For this review, take the finished solid that the model builds, in its own axes (mm). Face numbers are marked on the shaded views. A direction names the side the tool comes from. Give positions to 0.01 mm unless a question says otherwise; leave off trailing zeros. Order: outer loops, then holes, each group sorted by start corner. A loop starts at its lowest first (then second) coordinate and runs counter-clockwise, first axis right, second up.
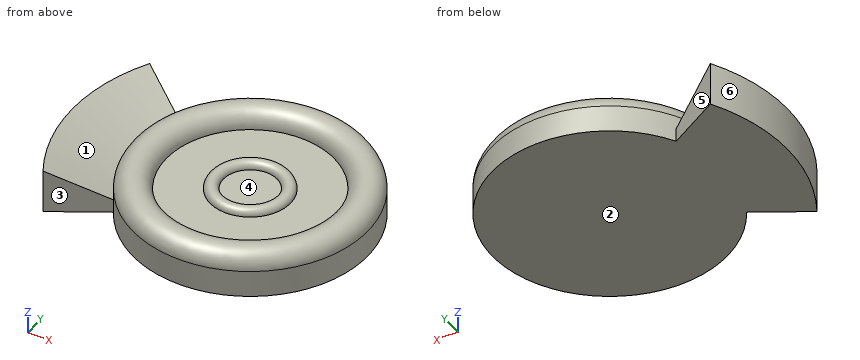
from build123d import *

# Parameters (mm, degrees)
F2_ANGLE = 60


with BuildPart() as f1:
    # F0 (on Front) → F1 (revolve)
    with BuildSketch(Plane.XZ):
        with BuildLine():
            Line((0, -8), (0, 0))
            Line((0, 0), (-8, 0))
            Line((-8, 0), (-12, 0))
            Line((-12, 0), (-25, 0))
            ThreePointArc((-25, 0), (-30, 5), (-35, 0))
            Line((-35, 0), (-35, -4))
            Line((-35, -4), (-35, -8))
            Line((-35, -8), (0, -8))
        make_face()
        with BuildLine():
            Line((-12, 0), (-8, 0))
            ThreePointArc((-8, 0), (-10, 2), (-12, 0))
        make_face()
    revolve(axis=Axis((0, 0, -4), (0, 0, -1)))

    # F0 (on Front) → F2 (revolve, symmetric)
    with BuildSketch(Plane.XZ) as f2_sk:
        Polygon((-53, -8), (-35, -8), (-35, -4), (-53, 5), align=None)
    revolve(axis=Axis((0, 0, -4), (0, 0, -1)), revolution_arc=F2_ANGLE / 2)
    revolve(f2_sk.sketch, axis=Axis((0, 0, -4), (0, 0, 1)), revolution_arc=F2_ANGLE / 2)


solid = f1.part
1) We need section A-A on x = 0. Give the boundary of the cut face in (y, z).
Answer sheet:
outline: (-35, -8) - (35, -8) - (35, 0) arc R5 ccw to (25, 0) - (12, 0) arc R2 ccw to (8, 0) - (-8, 0) arc R2 ccw to (-12, 0) - (-25, 0) arc R5 ccw to (-35, 0) - close
2) We need section B-B on y = 0. Give the boundary of the cut face in (x, z), then the cut area to 3 significant figures.
Answer sheet:
outline: (-53, -8) - (35, -8) - (35, 0) arc R5 ccw to (25, 0) - (12, 0) arc R2 ccw to (8, 0) - (-8, 0) arc R2 ccw to (-12, 0) - (-25, 0) arc R5 ccw to (-35, 0) - (-35, -4) - (-53, 5) - close
area: 804 mm2
3) Clearance check with flat-ended pins moving along their axes: pin 1 (6 mm diameter, centred on x = 19.5, z = 0, fed in from -Y); pin 2 (1 mm diameter, centred on x = -26, y = -3, fed in from +Z); pin 3 (2 mm diameter, centred on x = 4.5, y = -12.5, fed in from +Z); pin 4 (4 mm diameter, centred on x = 8.5, y = -27.5, fed in from +Z). State where each tip first meets the part, or that it passes through.
Answer sheet:
pin 1: stops at y = -30.87
pin 2: stops at z = 3.73
pin 3: stops at z = 0
pin 4: stops at z = 5
4) To check wall thickness, follow line 1 (X direction, y = 1.5, z = 0.5); line 2 (Y direction, x = 9, z = 0.25); line 3 (Z direction, x = 18.5, y = 14.5). State the ranges of each line that lie inside material, in increasing order.
Answer sheet:
line 1: x = -52.98 to -43.97, -34.94 to -24.98, -11.84 to -7.92, 7.92 to 11.84, 24.98 to 34.94
line 2: y = -33.82 to -23.33, -7.91 to 7.91, 23.33 to 33.82
line 3: z = -8 to 0
5) We need section C-C on z = -6. Give the boundary of the cut face in (x, y).
Answer sheet:
outline: (-45.9, -26.5) - (-30.31, -17.5) arc R35 ccw (long way) to (-30.31, 17.5) - (-45.9, 26.5) arc R53 ccw to start
6) Tool access review of the marked faces 4, 5 and 6: name each direction out of +Z, -Z, +X, -X, +Y, -Y from which nothing blocks a thin tool from reaching the whole face with its end or side.
Answer sheet:
face 4: +Z
face 5: +Z, -Z, +Y
face 6: +Z, -Z, -X
7) Draft analysis for pull direction Y (two halves, no side actions). For the marked faces 1, 2 and 3, state which applies: +Y half, -Y half, draft (parallel to the pull), parting line (faces both ways), or undercut.
Answer sheet:
face 1: undercut
face 2: draft
face 3: -Y half
